The listing builds one solid part. Answer for the finished solid, in the listing's coordinates (mm). Face numbers are marked on the shaded views. A direction names the side the tool comes from. Round coordinates to 2 decimals unless told otherwise and drop trailing zeros. Write each loop counter-clockwise with the first axis right and the second up, starting at its lowest first coordinate (ties: lowest second). Pieces come first, ordered by that corner, then holes. Notation, with made-up numbers: (17.5, 67.25) - (37.5, 67.25) arc R28 ccw to (37.5, 90.25) - close; hole circle Ø9 at (72, 66). An arc over 180 degrees is marked (long way). Answer in a Markdown table with one row per item.
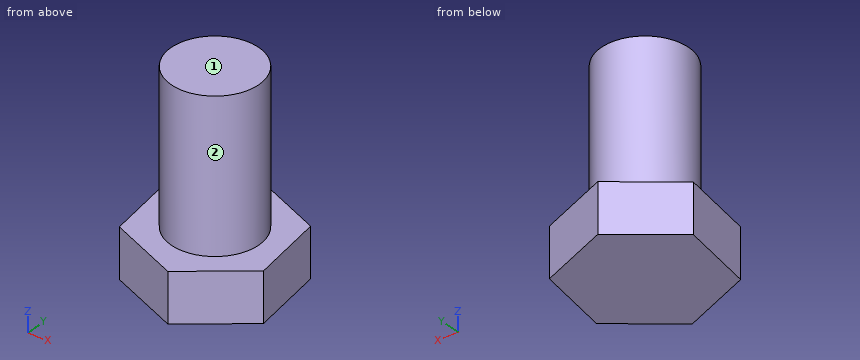
from build123d import *

# Parameters (mm, degrees)
F1_DEPTH = 2.667
F2_R     = 4.7625
F3_DEPTH = 16.256


with BuildPart() as f1:
    # F0 (on Top) → F1 (new body, symmetric)
    with BuildSketch(Plane.XY):
        Polygon((-1.245599, 8.065583), (-7.6078, 2.954071), (-6.3622, -5.111512), (1.245599, -8.065583), (7.6078, -2.954071), (6.3622, 5.111512), align=None)
    extrude(amount=F1_DEPTH, both=True)

    # F2 (on face) → F3 (join)
    with BuildSketch(Plane.XY.offset(2.667)):
        Circle(F2_R)
    extrude(amount=F3_DEPTH)


solid = f1.part
(1) Section C-C (z = 3.5) is taken. Give the vertices of the cut face in (x, y) (1 decimal).
Checked values:
| item | result |
|---|---|
| outline | circle Ø9.5 at (0, 0) |
(2) Section A-A (y = 0) is taken. Give the vertices of the cut face in (x, z).
Checked values:
| item | result |
|---|---|
| outline | (-7.15, -2.67) - (7.15, -2.67) - (7.15, 2.67) - (4.76, 2.67) - (4.76, 18.92) - (-4.76, 18.92) - (-4.76, 2.67) - (-7.15, 2.67) - close |
(3) Section B-B (x = -3) is taken. Give the vertices of the cut face in (y, z).
Checked values:
| item | result |
|---|---|
| outline | (-6.42, -2.67) - (6.66, -2.67) - (6.66, 2.67) - (3.7, 2.67) - (3.7, 18.92) - (-3.7, 18.92) - (-3.7, 2.67) - (-6.42, 2.67) - close |
(4) For the marked faces 1 and 2, determine the directions among +Z, -Z, +X, -X, +Y, -Y from which every point of the face is accessible in a straight line to the end or side of a thin tool.
Checked values:
| item | result |
|---|---|
| face 1 | +Z, +X, -X, +Y, -Y |
| face 2 | +Z |
(5) Find the intervals of material crossed by line 1 (Z direction, x = -4.25, y = 2.5); line 2 (X direction, y = 0.25, z = 12.5); line 3 (Y direction, x = 4, z = 12.25), in increasing order.
Checked values:
| item | result |
|---|---|
| line 1 | z = -2.67 to 2.67 |
| line 2 | x = -4.76 to 4.76 |
| line 3 | y = -2.58 to 2.58 |
(6) Section D-D (x = -6) is taken. Give the vertices of the cut face in (y, z).
Checked values:
| item | result |
|---|---|
| outline | (-5.25, -2.67) - (4.25, -2.67) - (4.25, 2.67) - (-5.25, 2.67) - close |
(7) A flat-ended cylindrical pin translates along its axis: pin 1 (3 mm diameter, centred on x = -5, z = 14.5, fed in from +Y). Find the tip coordinate at first contact, or state that the pin passes through.
Checked values:
| item | result |
|---|---|
| pin 1 | stops at y = 3.23 |
